from build123d import *

# Parameters (mm, degrees)
SKETCH001_W     = 23.25
SKETCH001_H     = 46.5
POCKET_DEPTH    = 16.001
POCKET001_DEPTH = 21
SKETCH003_W     = 4.5
SKETCH003_H     = 1
GROOVE_ANGLE    = 65
SKETCH004_W     = 6
SKETCH004_H     = 1
GROOVE001_ANGLE = 7
PAD_DEPTH       = 16
SKETCH006_W     = 8
SKETCH006_H     = 10
POCKET002_DEPTH = 16.001
SKETCH007_R     = 1.6
POCKET003_DEPTH = 26.251
POCKET004_DEPTH = 2.7
FILLET_R        = 7.999
SKETCH009_R     = 1.6
POCKET005_DEPTH = 16.001
PAD001_DEPTH    = 2


with BuildPart() as part:
    # Sketch → Revolution (revolve)
    with BuildSketch(Plane.XY):
        Polygon((0, -18.5), (10, -18.5), (10, -21.25), (14.5, -21.25), (14.5, -20.05), (16, -20.05), (16, -23.25), (14.5, -23.25), (10, -23.25), (0, -23.25), align=None)
    revolve(axis=Axis((0, 0, 0), (1, 0, 0)))

    # Sketch001 (on Face9 of Revolution) → Pocket (cut, through all)
    with BuildSketch(Plane.YZ.offset(16)):
        with Locations((-11.625, 0)):
            Rectangle(SKETCH001_W, SKETCH001_H)
    extrude(amount=-POCKET_DEPTH, mode=Mode.SUBTRACT)

    # Sketch002 (on Face2 of Pocket) → Pocket001 (cut)
    with BuildSketch(Plane.XZ):
        Polygon((0, 8.5), (10, 8.5), (10, 5.7), (6.3, 5.7), (6.3, -5.7), (10, -5.7), (10, -8.5), (0, -8.5), (0, -5.7), (3.5, -5.7), (3.5, 5.7), (0, 5.7), align=None)
    extrude(amount=-POCKET001_DEPTH, mode=Mode.SUBTRACT)

    # Sketch003 (on Face4 of Pocket001) → Groove (revolve, cut)
    with BuildSketch(Plane.XZ):
        with Locations((12.25, -21.75)):
            Rectangle(SKETCH003_W, SKETCH003_H)
    groove = revolve(axis=Axis((0, 0, 0), (1, 0, 0)), revolution_arc=GROOVE_ANGLE, mode=Mode.SUBTRACT)

    # Sketch004 (on Face4 of Groove) → Groove001 (revolve, cut)
    with BuildSketch(Plane.XZ):
        with Locations((12.25, -21.75)):
            Rectangle(SKETCH004_W, SKETCH004_H)
    groove001 = revolve(axis=Axis((0, 0, 0), (1, 0, 0)), revolution_arc=GROOVE001_ANGLE, mode=Mode.SUBTRACT)

    # Sketch005 (on Face12 of Groove001) → Pad (join)
    with BuildSketch(Plane(origin=(0, 0, 0), x_dir=(0, -1, 0), z_dir=(-1, 0, 0))):
        with BuildLine():
            ThreePointArc((0, 23.25), (-23.25, 0), (0, -23.25))
            Line((0, -36.25), (0, -23.25))
            Line((-26.25, -36.25), (0, -36.25))
            Line((-26.25, -36.25), (-26.25, 36.25))
            Line((-26.25, 36.25), (0, 36.25))
            Line((0, 36.25), (0, 23.25))
        make_face()
    extrude(amount=-PAD_DEPTH)

    # Sketch006 (on Face11 of Pad) → Pocket002 (cut, through all)
    with BuildSketch(Plane.YZ.offset(16)):
        with Locations((14, 31.25)):
            Rectangle(SKETCH006_W, SKETCH006_H)
        with Locations((14, -31.25)):
            Rectangle(SKETCH006_W, SKETCH006_H)
    extrude(amount=-POCKET002_DEPTH, mode=Mode.SUBTRACT)

    # Sketch007 (on Face40 of Pocket002) → Pocket003 (cut, through all)
    with BuildSketch(Plane(origin=(0, 26.25, 0), x_dir=(-1, 0, 0), z_dir=(0, 1, 0))):
        with Locations((-8, 31.25)):
            Circle(SKETCH007_R)
        with Locations((-8, -31.25)):
            Circle(SKETCH007_R)
    extrude(amount=-POCKET003_DEPTH, mode=Mode.SUBTRACT)

    # Sketch008 (on Face41 of Pocket003) → Pocket004 (cut)
    with BuildSketch(Plane(origin=(0, 26.25, 0), x_dir=(-1, 0, 0), z_dir=(0, 1, 0))):
        Polygon((-9.818653, 34.4), (-11.637307, 31.25), (-9.818653, 28.1), (-6.181347, 28.1), (-4.362693, 31.25), (-6.181347, 34.4), align=None)
        Polygon((-9.818653, -28.1), (-11.637307, -31.25), (-9.818653, -34.4), (-6.181347, -34.4), (-4.362693, -31.25), (-6.181347, -28.1), align=None)
    extrude(amount=-POCKET004_DEPTH, mode=Mode.SUBTRACT)

    # Mirrored: Groove001, Groove across XY
    add(groove001.mirror(Plane.XY), mode=Mode.SUBTRACT)
    add(groove.mirror(Plane.XY), mode=Mode.SUBTRACT)

    # Fillet
    fillet_edges = [part.edges().sort_by_distance(p)[0] for p in [
        (0, 22.125, 36.25),
        (0, 5, 36.25),
        (16, 5, 36.25),
        (16, 22.125, 36.25),
        (0, 22.125, -36.25),
        (0, 5, -36.25),
        (16, 22.125, -36.25),
        (16, 5, -36.25),
    ]]
    fillet(fillet_edges, radius=FILLET_R)

    # Sketch009 (on Face7 of Fillet) → Pocket005 (cut, through all)
    with BuildSketch(Plane.YZ.offset(16)):
        with Locations((20.007097, 22.008097)):
            Circle(SKETCH009_R)
        with Locations((20.007097, -22.008097)):
            Circle(SKETCH009_R)
    extrude(amount=-POCKET005_DEPTH, mode=Mode.SUBTRACT)

    # Sketch010 (on Face89 of Pocket005) → Pad001 (join)
    with BuildSketch(Plane.YZ.offset(10)):
        with BuildLine():
            ThreePointArc((18.439089, -1.5), (18.5, 0), (18.439089, 1.5))
            Line((18.439089, 1.5), (21.196993, 1.5))
            ThreePointArc((21.196993, -1.5), (21.25, 0), (21.196993, 1.5))
            Line((18.439089, -1.5), (21.196993, -1.5))
        make_face()
    extrude(amount=PAD001_DEPTH)


solid = part.part
Here's how the part is built. I have some questions about the finished solid (model axes, mm). A direction names the side the tool comes from. Give positions to 0.01 mm unless a question says otherwise; leave off trailing zeros. Order: outer loops, then holes, each group sorted by start corner. A loop starts at its lowest first (then second) coordinate and runs counter-clockwise, first axis right, second up. Notation, with made-up numbers: M -39,11 L 3,11 A21 cw 3,29 Z; hole C 7,62.5 d3. An arc over 180 degrees is marked long. Answer as a JSON object with one key per item and string values. Group by question number.
1) Suppose I cut it at C-C, the plane x = 5. Write out the boundary of the cut face in (y, z), plus the area to 3 significant figures.
2) On a 3-axis mill with a long thin cutter (end or side, diameter ignored), from which of +Z, -Z, +X, -X, +Y, -Y can I reach the whole of each face in a straight line? I mean faces 1 (the flat face through (10, 19, -4)), 2 (the flat face through (5, 19, -8.5)), 3 (the flat face through (8, 10, -29)), 4 (the flat face through (5.285, 24.919, 29.653)). Say none if no direction works.
3) I'm going to push flat-ended pins straight in: pin 1 Ø1.3 at (x, y) = (9, 25) entering from -Z; pin 2 Ø1 at (x, y) = (9, 20) entering from +Z; pin 3 Ø4 at (x, y) = (4, 12.5) entering from +Z. Where does each tip first touch, or does it pass through?
4) Please list where these lines run through material, in increasing order: L1, parallel to Z at x = 10.5, y = 24.25; L2, parallel to Y at x = 15, z = -29; L3, parallel to Z at x = 6, y = 17.25. Write a range as [from, to].
5) We'd pull the mould along Y, two halves only. Please class faces 5 (the flat face through (8, 18, -29)), 6 (the flat face through (11, 20, 1.5)), 7 (the cylindrical face through (1.8, 18.5, -0.1)): pulls with the +Y half, pulls with the -Y half, needs draft (parallel to the pull), parting line crosses it, or undercut.
6) Suppose I cut it at B-B, the plane z = 0. Write out the boundary of the cut face in (x, y), plus the area to 3 significant figures.
7) Suppose I cut it at A-A, the plane y = 4.5. Count the separate pieces of the cut face and the enclosed holes in it, plus the area to 3 significant figures.
8) Suppose I cut it at D-D, the plane y = 11. Write out the boundary of the cut face in (x, z).
Results found:
{
 "1": {"outline": "M 0,-35.67 L 10,-35.67 L 10,-26.25 L 18,-26.25 L 18,-35.67 L 26.25,-35.67 L 26.25,-32.35 L 23.55,-32.35 L 23.55,-30.15 L 26.25,-30.15 L 26.25,30.15 L 23.55,30.15 L 23.55,32.35 L 26.25,32.35 L 26.25,35.67 L 18,35.67 L 18,26.25 L 10,26.25 L 10,35.67 L 0,35.67 L 0,18.5 A18.5 cw 16.43,8.5 L 21,8.5 L 21,-8.5 L 16.43,-8.5 A18.5 cw 0,-18.5 Z; hole C 20.01,-22.01 d3.2; hole C 20.01,22.01 d3.2", "area": "1,100 mm²"},
 "2": {"face 1": "-Y", "face 2": "-X, -Y", "face 3": "-Z, +X, -X", "face 4": "+Y"},
 "3": {"pin 1": "z = -36.24", "pin 2": "z = 36.23", "pin 3": "z = 26.25"},
 "4": {"L1": "[-35.85, -33.22], [-29.28, 29.28], [33.22, 35.85]", "L2": "[0, 10], [18, 26.25]", "L3": "[-26.25, -8.5], [8.5, 26.25]"},
 "5": {"face 5": "undercut", "face 6": "needs draft", "face 7": "pulls with the -Y half"},
 "6": {"outline": "M 0,18.5 L 3.5,18.5 L 3.5,21 L 6.3,21 L 6.3,18.5 L 12,18.5 L 12,21.25 L 14.5,21.25 L 14.5,20.05 L 16,20.05 L 16,26.25 L 0,26.25 Z", "area": "108 mm²"},
 "7": {"separate pieces": "2", "enclosed holes": "2", "area": "475 mm²"},
 "8": {"outline": "M 0,-26.25 L 16,-26.25 L 16,-16.76 L 14.5,-16.76 L 14.5,-19.34 L 10,-19.34 L 10,-14.87 L 0,-14.87 Z; M 0,14.87 L 10,14.87 L 10,19.34 L 14.5,19.34 L 14.5,16.76 L 16,16.76 L 16,26.25 L 0,26.25 Z"}
}
